from build123d import *

# Parameters (mm, degrees)
SKETCH_1_W          = 15.4
SKETCH_1_H          = 22.4
EXTRUDE_2_DEPTH     = 3
EXTRUDE_3_DEPTH     = 10
EXTRUDE_3_2_DEPTH   = 10
EXTRUDE_4_DEPTH     = 40
SKETCH_3_R          = 1.6
CUT_EXTRUDE_2_DEPTH = 31.8
SKETCH_10_R         = 3
CUT_EXTRUDE_7_DEPTH = 2
SKETCH_11_R         = 3
CUT_EXTRUDE_8_DEPTH = 2
SKETCH_12_W         = 15.4
SKETCH_12_H         = 15.4
CUT_EXTRUDE_9_DEPTH = 4


with BuildPart() as part:
    # Sketch 1 → Extrude 2 (new body)
    with BuildSketch(Plane(origin=(0, 0, 0), x_dir=(1, 0, 0), z_dir=(0, 1, 0))):
        Rectangle(SKETCH_1_W, SKETCH_1_H)
    extrude(amount=EXTRUDE_2_DEPTH)



with BuildPart() as body_2:
    # Sketch 1_4 → Extrude 3 (new body)
    with BuildSketch(Plane(origin=(0, 0, 0), x_dir=(1, 0, 0), z_dir=(0, 1, 0))):
        Polygon((7.7, -11.2), (7.7, -7.7), (0, -7.7), (-4.7, -7.7), (-7.7, -7.7), (-7.7, -11.2), align=None)
    extrude(amount=EXTRUDE_3_DEPTH)


with BuildPart() as body_3:
    # Sketch 1_4 → Extrude 3 2 (new body)
    with BuildSketch(Plane(origin=(0, 0, 0), x_dir=(1, 0, 0), z_dir=(0, 1, 0))):
        Polygon((-7.7, 7.7), (0, 7.7), (7.7, 7.7), (7.7, 11.2), (-7.7, 11.2), align=None)
    extrude(amount=EXTRUDE_3_2_DEPTH)


with BuildPart() as part_1:
    add(part.part)

    add(body_2.part)  # Extrude 4 merges body 2

    add(body_3.part)  # Extrude 4 merges body 3
    # Sketch 1_5 → Extrude 4 (add)
    with BuildSketch(Plane(origin=(0, 0, 0), x_dir=(1, 0, 0), z_dir=(0, 1, 0))):
        Polygon((-7.7, 0), (-7.7, 7.7), (-7.7, 11.2), (-11.2, 11.2), (-11.2, -11.2), (-7.7, -11.2), (-7.7, -7.7), align=None)
        Polygon((7.7, 11.2), (7.7, 7.7), (7.7, 0), (7.7, -7.7), (7.7, -11.2), (11.2, -11.2), (11.2, 11.2), align=None)
        Polygon((7.7, -11.2), (7.7, -7.7), (0, -7.7), (-4.7, -7.7), (-7.7, -7.7), (-7.7, -11.2), align=None)
        Polygon((-7.7, 7.7), (0, 7.7), (7.7, 7.7), (7.7, 11.2), (-7.7, 11.2), align=None)
    extrude(amount=EXTRUDE_4_DEPTH)

    # Sketch 3 → Cut-Extrude 2 (cut, through all)
    with BuildSketch(Plane(origin=(0, 0, -19.6), x_dir=(-1, 0, 0), z_dir=(0, 0, -1))):
        with Locations((0, 10)):
            Circle(SKETCH_3_R)
        with Locations((0, 30)):
            Circle(SKETCH_3_R)
    extrude(amount=-CUT_EXTRUDE_2_DEPTH, mode=Mode.SUBTRACT)

    # Sketch 10 → Cut-Extrude 7 (cut)
    with BuildSketch(Plane(origin=(0, 0, -11.2), x_dir=(-1, 0, 0), z_dir=(0, 0, -1))):
        with Locations((0, 30)):
            Circle(SKETCH_10_R)
        with Locations((0, 10)):
            Circle(SKETCH_10_R)
    extrude(amount=-CUT_EXTRUDE_7_DEPTH, mode=Mode.SUBTRACT)

    # Sketch 11 → Cut-Extrude 8 (cut)
    with BuildSketch(Plane.XY.offset(11.2)):
        with Locations((0, 30)):
            Circle(SKETCH_11_R)
        with Locations((0, 10)):
            Circle(SKETCH_11_R)
    extrude(amount=-CUT_EXTRUDE_8_DEPTH, mode=Mode.SUBTRACT)

    # Sketch 12 → Cut-Extrude 9 (cut, through all)
    with BuildSketch(Plane(origin=(0, 3, 0), x_dir=(1, 0, 0), z_dir=(0, 1, 0))):
        Rectangle(SKETCH_12_W, SKETCH_12_H)
    extrude(amount=-CUT_EXTRUDE_9_DEPTH, mode=Mode.SUBTRACT)


solid = part_1.part
Check sheet for the modelled part. Datum: model origin and axes. Units: mm. A direction names the side the tool comes from. Round coordinates to 2 decimals unless told otherwise and drop trailing zeros. Loops run counter-clockwise (first coordinate to the right, second up) from the corner with the lowest first, then second, coordinate; pieces in that order, holes last. Notation, with made-up numbers: (75, -25) - (79, -25) arc R26 ccw to (79, -2) - close; hole circle Ø7 at (41, -1). An arc over 180 degrees is marked (long way). Answer as CSV lines item,"result". Start each with the question number.
Item 1: Release check for a two-part mould opening along Y. For faces 4 (the flat face through (0, 20, 11.2)), 5 (the flat face through (-10, 40, 0)), 6 (the cylindrical face through (0.35, 8.44, -8.46)), 7 (the cylindrical face through (0.208, 31.586, 8.439)) record: +Y half, -Y half, draft (parallel to the pull), parting line (faces both ways), or undercut.
Item 2: Set-up check for faces 1 (the cylindrical face through (-2.21, 32.03, 10.21)), 2 (the cylindrical face through (3, 10, -10)), 3 (the flat face through (7.7, 20, 0)): record each of +Z, -Z, +X, -X, +Y, -Y from which the full face is reachable in a straight line by a thin tool's end or side.
Item 3: Section check B-B (y = 10). Record the boundary of the cut face in (x, z), and give its area (3 significant figures).
Item 4: Section check D-D (y = 24). Record the boundary of the cut face in (x, z).
Item 5: Depth check by flat-ended pin: P1, Ø4, axis at x = 0, y = 10, coming from the -Z side; P2, Ø3, axis at x = 0, y = 30, coming from the -Z side; P3, Ø9.5, axis at x = 0, y = 30, coming from the +Z side; P4, Ø5, axis at x = 0, y = 10, coming from the +Z side. Enter the tip coordinate at first touch or a pass-through.
Item 6: Section check C-C (x = 4). Record the boundary of the cut face in (y, z), and give its area (3 significant figures).
Item 7: Section check A-A (z = 6.5). Record the boundary of the cut face in (x, y), and give its area (3 significant figures).
Item 8: Scan lines: line 1 (Y direction, x = 0, z = -8.2); line 2 (Y direction, x = 0, z = 9.85); line 3 (Z direction, x = 5, y = 32.5). Record each from-to range of solid material in increasing order. Write a range as [from, to].
Report:
1,face 4,"draft"
1,face 5,"+Y half"
1,face 6,"undercut"
1,face 7,"undercut"
2,face 1,"+Z"
2,face 2,"-Z"
2,face 3,"+Y, -Y"
3,outline,"(-11.2, -11.2) - (-3, -11.2) - (-3, -9.2) - (-1.6, -9.2) - (-1.6, -7.7) - (-7.7, -7.7) - (-7.7, 7.7) - (-1.6, 7.7) - (-1.6, 9.2) - (-3, 9.2) - (-3, 11.2) - (-11.2, 11.2) - close; (1.6, -9.2) - (3, -9.2) - (3, -11.2) - (11.2, -11.2) - (11.2, 11.2) - (3, 11.2) - (3, 9.2) - (1.6, 9.2) - (1.6, 7.7) - (7.7, 7.7) - (7.7, -7.7) - (1.6, -7.7) - close"
3,area,"231 mm2"
4,outline,"(-11.2, -11.2) - (11.2, -11.2) - (11.2, 11.2) - (-11.2, 11.2) - close; hole (-7.7, -7.7) - (7.7, -7.7) - (7.7, 7.7) - (-7.7, 7.7) - close"
5,P1,"stops at z = -9.2"
5,P2,"passes through"
5,P3,"stops at z = 11.2"
5,P4,"stops at z = 9.2"
6,outline,"(0, -11.2) - (40, -11.2) - (40, -7.7) - (0, -7.7) - close; (0, 7.7) - (40, 7.7) - (40, 11.2) - (0, 11.2) - close"
6,area,"280 mm2"
7,outline,"(-11.2, 0) - (-7.7, 0) - (-7.7, 40) - (-11.2, 40) - close; (7.7, 0) - (11.2, 0) - (11.2, 40) - (7.7, 40) - close"
7,area,"280 mm2"
8,line 1,"y = [0, 8.4], [11.6, 28.4], [31.6, 40]"
8,line 2,"y = [0, 7], [13, 27], [33, 40]"
8,line 3,"z = [-11.2, -7.7], [7.7, 11.2]"
